from build123d import *

# Parameters (mm, degrees)
F0_W     = 200
F0_H     = 140
F0_W_2   = 125.75
F0_H_2   = 85
F1_DEPTH = 7.5
F3_D     = 8
F3_DEPTH = 12
F4_DEPTH = 15


with BuildPart() as f1:
    # F0 (on Front) → F1 (new body)
    with BuildSketch(Plane.XZ):
        with Locations((-116.173333, 64.000176)):
            Rectangle(F0_W, F0_H)
        with Locations((-116.173333, 64.000176)):
            Rectangle(F0_W_2, F0_H_2, mode=Mode.SUBTRACT)
    extrude(amount=F1_DEPTH)

    # F3
    with Locations(Plane.XZ.offset(7.5)):
        with Locations((-39.681189, 21.607968), (-192.181189, 21.607968), (-192.181189, 107.607968), (-39.681189, 107.607968)):
            Hole(F3_D / 2, depth=F3_DEPTH)

    # F0 (on Front) → F4 (join)
    with BuildSketch(Plane.XZ):
        with Locations((-116.173333, 64.000176)):
            Rectangle(F0_W_2, F0_H_2)
    extrude(amount=F4_DEPTH)


solid = f1.part
Design review of the part built by this model. Coordinates are the model's own, in mm. A direction names the side the tool comes from. Round coordinates to 2 decimals unless told otherwise and drop trailing zeros. Write each loop counter-clockwise with the first axis right and the second up, starting at its lowest first coordinate (ties: lowest second). Pieces come first, ordered by that corner, then holes. Notation, with made-up numbers: M 57,10.5 L 84,10.5 A3 ccw 84,14.5 Z; hole C -4.75,-15 d4. An arc over 180 degrees is marked long. One line per item, written item: value. Start each with the question number.
1. Take a section at A-A on z = 76.5. State the section outline as (x, y) points, then the cut area to 3 significant figures.
2. Take a section at C-C on y = -10. State the section outline as (x, z) points.
3. Clearance check with flat-ended pins moving along their axes: P1, Ø6, axis at x = -115, y = -12.5, coming from the -Z side; P2, Ø5, axis at y = -11.5, z = 40.5, coming from the -X side; P3, Ø6, axis at y = -12, z = 50, coming from the +X side. State where each tip first meets the part, or that it passes through.
4. Draft analysis for pull direction Z (two halves, no side actions). For faces 5 (the face through (-53.298, -11, 63)), 6 (the face through (-189.23, -3.7, 24.31)), 7 (the face through (-118, -4, 134)), state which applies: pulls with the +Z half, pulls with the -Z half, needs draft (parallel to the pull), parting line crosses it, or undercut.
5. Take a section at B-B on x = -84.5. State the section outline as (y, z) points.
6. For faces 1 (the face through (-179.048, -11, 63)), 2 (the face through (-117, -15, 65)), 3 (the face through (-117, -11, 21.5)), 4 (the face through (-117, -11, 106.5)), list the 3-axis set-ups (+Z, -Z, +X, -X, +Y, -Y) from which the entire face can be reached by the end or side of a thin tool; tool diameter is ignored.
7. Take a section at D-D on x = -199. State the section outline as (y, z) points, then the cut area to 3 significant figures.
8. To check wall thickness, follow probe 1 along X at (y, z) = (-4.5, 110.5); probe 2 along Y at (x, z) = (-88.5, 5.5); probe 3 along Z at (x, y) = (-155, -12.5). State the ranges of each line that lie inside material, in increasing order. Write a range as from..to.
Computed:
1. outline: M -216.17,-7.5 L -179.05,-7.5 L -179.05,-15 L -53.3,-15 L -53.3,-7.5 L -16.17,-7.5 L -16.17,0 L -216.17,0 Z
1. area: 2,440 mm²
2. outline: M -179.05,21.5 L -53.3,21.5 L -53.3,106.5 L -179.05,106.5 Z
3. P1: stops at z = 21.5
3. P2: stops at x = -179.05
3. P3: stops at x = -53.3
4. face 5: needs draft
4. face 6: undercut
4. face 7: pulls with the +Z half
5. outline: M -15,21.5 L -7.5,21.5 L -7.5,-6 L 0,-6 L 0,134 L -7.5,134 L -7.5,106.5 L -15,106.5 Z
6. face 1: +Z, -Z, -X, -Y
6. face 2: +Z, -Z, +X, -X, -Y
6. face 3: -Z, +X, -X, -Y
6. face 4: +Z, +X, -X, -Y
7. outline: M -7.5,-6 L 0,-6 L 0,134 L -7.5,134 Z
7. area: 1,050 mm²
8. probe 1: x = -216.17..-194.94, -189.42..-42.44, -36.92..-16.17
8. probe 2: y = -7.5..0
8. probe 3: z = 21.5..106.5
